Study the drawing (mm; zero at the part's minimum x, y, z) and answer. Give positions to 0.01 mm unless a question says otherwise; leave off trailing zeros. Order: outer loops, then holes, each group sorted by start corner. A loop starts at its lowest first (then second) coordinate and runs counter-clockwise, first axis right, second up. Notation, with made-up numbers: (-37.75, 4.5) - (-3.75, 4.5) arc R29 ccw to (-3.75, 37.5) - close; hole circle Ø2 at (74.25, 44.5). An arc over 180 degrees is marked (long way). Return JSON: item names as keys, results as strings.
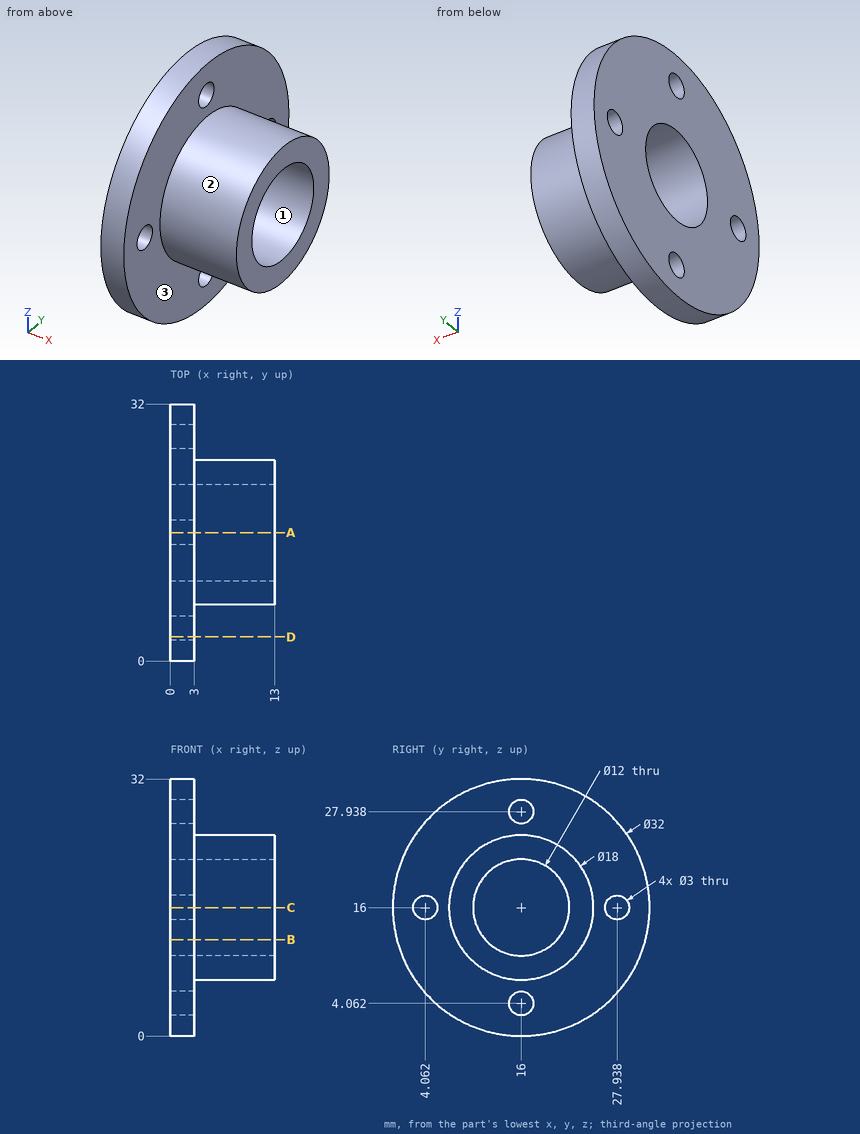
Q1. A cutting plane is placed at B-B (z = 12). Write down the section's boundary in (x, y).
Values:
{"outline": "(0, 0.51) - (3, 0.51) - (3, 7.94) - (13, 7.94) - (13, 11.53) - (0, 11.53) - close; (0, 20.47) - (13, 20.47) - (13, 24.06) - (3, 24.06) - (3, 31.49) - (0, 31.49) - close"}
Q2. Determine the mould class of the marked faces 1, 2 and 3 for opening direction Z: released by +Z, released by -Z, zero draft, split by the parting line, or undercut.
Values:
{"face 1": "undercut", "face 2": "split by the parting line", "face 3": "zero draft"}
Q3. A cutting plane is placed at D-D (y = 3). Write down the section's boundary in (x, z).
Values:
{"outline": "(0, 6.67) - (3, 6.67) - (3, 14.94) - (0, 14.94) - close; (0, 17.06) - (3, 17.06) - (3, 25.33) - (0, 25.33) - close"}
Q4. Given pin 1 (5 mm diameter, centred on y = 27.938, z = 16, fed in from -X); pin 2 (1.5 mm diameter, centred on x = 3, y = 20.5, fed in from +Z); pin 3 (1 mm diameter, centred on x = 2.5, z = 4.5, fed in from -Y); pin 4 (2 mm diameter, centred on x = 5.5, z = 10.5, fed in from -Y), each flat-ended and moving along its own axis, determine where each tip first touches the part or whether it passes through.
Values:
{"pin 1": "stops at x = 0", "pin 2": "stops at z = 31.55", "pin 3": "stops at y = 4.38", "pin 4": "stops at y = 8.21"}
Q5. Consider L1, parallel to X at y = 6.5, z = 14.5; L2, parallel to Z at x = 2.5, y = 15; L3, parallel to Z at x = 11, y = 11. Determine where each line is inside the solid, lowest interval first.
Values:
{"L1": "x = 0 to 3", "L2": "z = 0.03 to 2.94, 5.18 to 10.08, 21.92 to 26.82, 29.06 to 31.97", "L3": "z = 8.52 to 12.68, 19.32 to 23.48"}
Q6. A cutting plane is placed at A-A (y = 16). Write down the section's boundary in (x, z).
Values:
{"outline": "(0, 0) - (3, 0) - (3, 2.56) - (0, 2.56) - close; (0, 5.56) - (3, 5.56) - (3, 7) - (13, 7) - (13, 10) - (0, 10) - close; (0, 22) - (13, 22) - (13, 25) - (3, 25) - (3, 26.44) - (0, 26.44) - close; (0, 29.44) - (3, 29.44) - (3, 32) - (0, 32) - close"}
